```python
from build123d import *

# Parameters (mm, degrees)
SKETCH_1_W             = 36
SKETCH_1_H             = 7
SKETCH_1_R             = 0.5
EXTRUDE_1_DEPTH        = 3.5
HOLE_WIZARD_M4_1_D     = 3.3
HOLE_WIZARD_M4_1_DEPTH = 22.1
HOLE_WIZARD_M4_1_TIP   = 0.991420021
HOLE_WIZARD_M4_2_D     = 3.3
HOLE_WIZARD_M4_2_DEPTH = 22.1
HOLE_WIZARD_M4_2_TIP   = 0.991420021


with BuildPart() as part:
    # 草图1 → 凸台-拉伸1 (new body, symmetric)
    with BuildSketch(Plane.XY):
        Rectangle(SKETCH_1_W, SKETCH_1_H)
        with Locations((-15, 0)):
            Circle(SKETCH_1_R, mode=Mode.SUBTRACT)
        with Locations((15, 0)):
            Circle(SKETCH_1_R, mode=Mode.SUBTRACT)
    extrude(amount=EXTRUDE_1_DEPTH, both=True)

    # M4 螺纹孔1
    with Locations(Plane.XY.offset(3.5)):
        with Locations((-15, 0), (15, 0)):
            Hole(HOLE_WIZARD_M4_1_D / 2, depth=HOLE_WIZARD_M4_1_DEPTH)
            with Locations((0, 0, -(HOLE_WIZARD_M4_1_DEPTH + HOLE_WIZARD_M4_1_TIP / 2))):  # 118° drill point
                Cone(0, HOLE_WIZARD_M4_1_D / 2, HOLE_WIZARD_M4_1_TIP, mode=Mode.SUBTRACT)

    # M4 螺纹孔2
    with Locations(Plane(origin=(0, 3.5, 0), x_dir=(1, 0, 0), z_dir=(0, 1, 0))):
        with Locations((0, 0)):
            Hole(HOLE_WIZARD_M4_2_D / 2, depth=HOLE_WIZARD_M4_2_DEPTH)
            with Locations((0, 0, -(HOLE_WIZARD_M4_2_DEPTH + HOLE_WIZARD_M4_2_TIP / 2))):  # 118° drill point
                Cone(0, HOLE_WIZARD_M4_2_D / 2, HOLE_WIZARD_M4_2_TIP, mode=Mode.SUBTRACT)


solid = part.part
```
Design review of the part built by this model. Coordinates are the model's own, in mm. Give positions to 0.01 mm unless a question says otherwise; leave off trailing zeros. Write each loop counter-clockwise with the first axis right and the second up, starting at its lowest first coordinate (ties: lowest second). Pieces come first, ordered by that corner, then holes. Notation, with made-up numbers: (65, 22.5) - (96, 22.5) arc R27 cw to (96, 50.5) - close; hole circle Ø10 at (62, -31.5). An arc over 180 degrees is marked (long way). Return JSON: item names as keys, results as strings. Group by question number.
(1) We need section C-C, the plane x = 15. Give the boundary of the cut face in (y, z).
(2) To check wall thickness, follow probe 1 along Z at (x, y) = (0, -1); probe 2 along X at (y, z) = (1.5, 3). State the ranges of each line that lie inside material, in increasing order.
(3) Mouldability with a two-part tool opening along X and no side actions: class faces 1 (the flat face through (0, 3.5, 2)), 2 (the flat face through (-18, 0, 0)), 3 (the flat face through (18, 0, 0)), 4 (the cylindrical face through (1.216, -0.049, -1.115)) as +X half, -X half, draft (parallel to the pull), parting line (faces both ways), or undercut.
(4) We need section D-D, the plane z = -2.5. Give the boundary of the cut face in (x, y), then the cut area to 3 significant figures.
(5) We need section A-A, the plane y = 0. Give the boundary of the cut face in (x, z), then the cut area to 3 significant figures.
(6) We need section B-B, the plane z = 0. Give the boundary of the cut face in (x, y).
Reported:
{
 "1": {"outline": "(-3.5, -3.5) - (-1.65, -3.5) - (-1.65, 3.5) - (-3.5, 3.5) - close; (1.65, -3.5) - (3.5, -3.5) - (3.5, 3.5) - (1.65, 3.5) - close"},
 "2": {"probe 1": "z = -3.5 to -1.65, 1.65 to 3.5", "probe 2": "x = -18 to -15.69, -14.31 to 14.31, 15.69 to 18"},
 "3": {"face 1": "draft", "face 2": "-X half", "face 3": "+X half", "face 4": "undercut"},
 "4": {"outline": "(-18, -3.5) - (18, -3.5) - (18, 3.5) - (-18, 3.5) - close; hole circle Ø3.3 at (-15, 0); hole circle Ø3.3 at (15, 0)", "area": "235 mm2"},
 "5": {"outline": "(-18, -3.5) - (-16.65, -3.5) - (-16.65, 3.5) - (-18, 3.5) - close; (-13.35, -3.5) - (13.35, -3.5) - (13.35, 3.5) - (-13.35, 3.5) - close; (16.65, -3.5) - (18, -3.5) - (18, 3.5) - (16.65, 3.5) - close; hole circle Ø3.3 at (0, 0)", "area": "197 mm2"},
 "6": {"outline": "(-18, -3.5) - (-1.65, -3.5) - (-1.65, 3.5) - (-18, 3.5) - close; (1.65, -3.5) - (18, -3.5) - (18, 3.5) - (1.65, 3.5) - close; hole circle Ø3.3 at (-15, 0); hole circle Ø3.3 at (15, 0)"}
}
